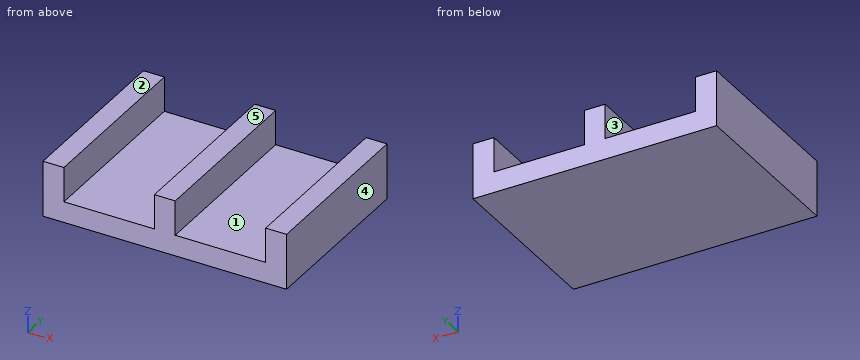
```python
from build123d import *

# Parameters (mm, degrees)
F0_W     = 35
F0_H     = 25
F1_DEPTH = 3
F2_W     = 1.5
F2_H     = 12.5
F3_DEPTH = 5
F4_W     = 3
F4_H     = 25
F5_DEPTH = 5
F6_W     = 3
F6_H     = 25
F7_DEPTH = 5


with BuildPart() as f1:
    # F0 (on Top) → F1 (new body)
    with BuildSketch(Plane.XY):
        with Locations((41.165313, -53.700294)):
            Rectangle(F0_W, F0_H)
    extrude(amount=F1_DEPTH)

    # F2 (on face) → F3 (join)
    with BuildSketch(Plane.XY.offset(3)):
        with Locations((40.415313, -47.450294)):
            Rectangle(F2_W, F2_H)
        with Locations((40.415313, -59.950294)):
            Rectangle(F2_W, F2_H)
        with Locations((41.915313, -47.450294)):
            Rectangle(F2_W, F2_H)
        with Locations((41.915313, -59.950294)):
            Rectangle(F2_W, F2_H)
    extrude(amount=F3_DEPTH)

    # F4 (on face) → F5 (join)
    with BuildSketch(Plane.XY.offset(3)):
        with Locations((25.165313, -53.700294)):
            Rectangle(F4_W, F4_H)
    extrude(amount=F5_DEPTH)

    # F6 (on face) → F7 (join)
    with BuildSketch(Plane.XY.offset(3)):
        with Locations((57.165313, -53.700294)):
            Rectangle(F6_W, F6_H)
    extrude(amount=F7_DEPTH)


solid = f1.part
```
The listing builds one solid part. Answer for the finished solid, in the listing's coordinates (mm). Face numbers are marked on the shaded views. A direction names the side the tool comes from. Give positions to 0.01 mm unless a question says otherwise; leave off trailing zeros. Write each loop counter-clockwise with the first axis right and the second up, starting at its lowest first coordinate (ties: lowest second). Pieces come first, ordered by that corner, then holes. Notation, with made-up numbers: M 87,-39.5 L 139,-39.5 A10 ccw 139,-30.5 Z; hole C 67,41 d9. An arc over 180 degrees is marked long. Write each question's results on one line, items separated by ' | '.
Q1. A flat-ended cylindrical pin translates along its axis: P1, Ø6.5, axis at x = 35, y = -51, coming from the +Z side. Find the tip coordinate at first contact, or state that the pin passes through.
Output values:
P1: z = 3
Q2. Section B-B, the plane y = -42.75 is taken. Write down the section's boundary in (x, z).
Output values:
outline: M 23.67,0 L 58.67,0 L 58.67,8 L 55.67,8 L 55.67,3 L 42.67,3 L 42.67,8 L 39.67,8 L 39.67,3 L 26.67,3 L 26.67,8 L 23.67,8 Z
Q3. Section C-C, the plane x = 35.5 is taken. Write down the section's boundary in (y, z).
Output values:
outline: M -66.2,0 L -41.2,0 L -41.2,3 L -66.2,3 Z
Q4. Section A-A, the plane z = 6.25 is taken. Write down the section's boundary in (x, y).
Output values:
outline: M 23.67,-66.2 L 26.67,-66.2 L 26.67,-41.2 L 23.67,-41.2 Z; M 39.67,-66.2 L 42.67,-66.2 L 42.67,-41.2 L 39.67,-41.2 Z; M 55.67,-66.2 L 58.67,-66.2 L 58.67,-41.2 L 55.67,-41.2 Z
Q5. Consider L1, parallel to X at y = -64.5, z = 7.5; L2, parallel to Z at x = 31, y = -51.25. Determine where each line is inside the solid, lowest interval first. Write a range as from..to.
Output values:
L1: 23.67..26.67, 39.67..42.67, 55.67..58.67 | L2: 0..3
Q6. For a pull along X with two mould halves and no side action, classify the marked faces 3, 4 and 5 as released by +X, released by -X, zero draft, split by the parting line, or undercut.
Output values:
face 3: undercut | face 4: released by +X | face 5: zero draft
Q7. A tool of negligible diameter and unlimited length cuts with its end or side. For the marked faces 1 and 2, from which of +Z, -Z, +X, -X, +Y, -Y can it reach the whole face along a straight path? Write none if from no direction.
Output values:
face 1: +Z, +Y, -Y | face 2: +Z, +X, -X, +Y, -Y
